```python
from build123d import *
from build123d.topology import SkipClean

# Parameters (mm, degrees)
SKETCH2_R           = 15
BOSS_EXTRUDE1_DEPTH = 170
BOSS_EXTRUDE2_START = 15.982197964
BOSS_EXTRUDE2_DEPTH = 15.982197964
SKETCH5_R           = 3
CUT_EXTRUDE1_DEPTH  = 19
FILLET5_R           = 10


with BuildPart() as part:
    # Sketch2 → Boss-Extrude1 (new body)
    with BuildSketch(Plane(origin=(0, 0, 0), x_dir=(1, 0, 0), z_dir=(0, 1, 0))):
        with Locations(Location((0, 0, 0), (0, 0, 270))):
            Circle(SKETCH2_R)
    extrude(amount=BOSS_EXTRUDE1_DEPTH)

    # Sketch3 → Boss-Extrude2 (add)
    with SkipClean():  # the faces are left unmerged after this step: merging them gives an invalid solid
        with BuildSketch(Plane.XZ.offset(BOSS_EXTRUDE2_START)):
            with BuildLine():
                Line((-15, 0), (15, 0))
                ThreePointArc((15, 0), (0, 15), (-15, 0))
            make_face()
        extrude(amount=-BOSS_EXTRUDE2_DEPTH)

    # Sketch5 → Cut-Extrude1 (cut)
    with SkipClean():  # the faces are left unmerged after this step: merging them gives an invalid solid
        with BuildSketch(Plane(origin=(0, 0, 0), x_dir=(-1, 0, 0), z_dir=(0, 0, -1))):
            with Locations((0, -8.732260388)):
                Circle(SKETCH5_R)
        extrude(amount=-CUT_EXTRUDE1_DEPTH, mode=Mode.SUBTRACT)

    # Fillet5
    # the kernel refuses this fillet: 10 mm, written as the material it takes off along each edge
    with BuildSketch(Plane(origin=(0, -15.982197964, 0), x_dir=(0.0031415874858799616, 0, -0.9999950652018581), z_dir=(-0.9999950652018581, 0, -0.0031415874858799616))) as fillet5_piece_1:
        with BuildLine():
            CenterArc((15 - FILLET5_R, -FILLET5_R), FILLET5_R, 0, 90)
            Line((15 - FILLET5_R, 0), (15, 0))
            Line((15, 0), (15, -FILLET5_R))
        make_face()
    revolve(axis=Axis((0, -15.982197964, 0), (0, -1, 0)), revolution_arc=359.64, mode=Mode.SUBTRACT)


solid = part.part
```
Check sheet for the modelled part. Datum: model origin and axes. Units: mm. Give positions to 0.01 mm unless a question says otherwise; leave off trailing zeros. Order: outer loops, then holes, each group sorted by start corner. A loop starts at its lowest first (then second) coordinate and runs counter-clockwise, first axis right, second up. Notation, with made-up numbers: (18, -3.5) -> (40, -3.5) arc R6 ccw to (40, 7.5) -> close; hole circle Ø8 at (81, 82). An arc over 180 degrees is marked (long way). Return JSON: item names as keys, results as strings.
1. Cross-section at B-B, the plane z = -8.5. Record the cut outline in (x, y), plus the area to 3 significant figures.
From the geometry:
{"outline": "(-12.36, 0) -> (12.36, 0) -> (12.36, 170) -> (-12.36, 170) -> close", "area": "4,200 mm^2"}
2. Mould release check, pull along Z, two halves, no side actions. Record for faces 1 (the flat face through (0, -5, 0)), 2 (the flat face through (0, 0, -6)): +Z half, -Z half, draft (parallel to the pull), parting line (faces both ways), or undercut.
From the geometry:
{"face 1": "-Z half", "face 2": "draft"}
3. Go/stop test with flat-tipped pins: P1, Ø5, axis at y = 111, z = -6.5, coming from the +X side; P2, Ø3, axis at x = 6, y = 60.5, coming from the -Z side; P3, Ø5, axis at x = 1.5, y = -9, coming from the -Z side. Record where each tip stops, or that it passes through.
From the geometry:
{"P1": "x = 14.46", "P2": "z = -14.31", "P3": "z = 0"}
4. Cross-section at C-C, the plane y = -2. Record the cut outline in (x, z).
From the geometry:
{"outline": "(-15, 0) -> (15, 0) arc R15 ccw to start"}
5. Material ranges on probe 1 along Y at (x, z) = (0, 5); probe 2 along Y at (x, z) = (-3, -12); probe 3 along Y at (x, z) = (0, 9.25), recorded low to high. Write a range as [from, to].
From the geometry:
{"probe 1": "[-15.98, -11.73], [-5.73, 170]", "probe 2": "[0, 170]", "probe 3": "[-15.03, -11.73], [-5.73, 170]"}
6. Cross-section at A-A, the plane y = 32.5. Record the cut outline in (x, z).
From the geometry:
{"outline": "circle Ø30 at (0, 0)"}
